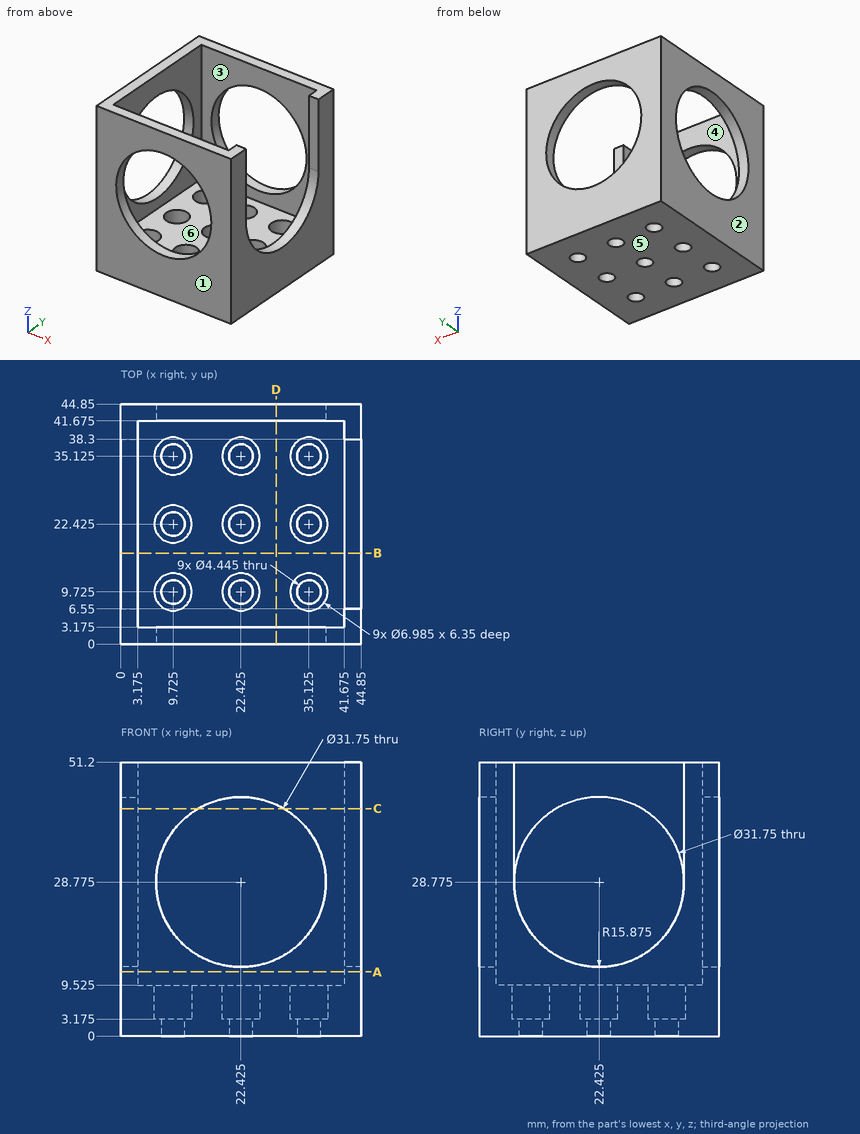
Geometry check sheet. Reference: drawing and pictorial views, mm from the part's lowest x, y, z. A direction names the side the tool comes from. Round coordinates to 2 decimals unless told otherwise and drop trailing zeros. Loops run counter-clockwise (first coordinate to the right, second up) from the corner with the lowest first, then second, coordinate; pieces in that order, holes last. Notation, with made-up numbers: (66.5, 68) - (124.5, 68) arc R36 cw to (124.5, 104) - close; hole circle Ø2 at (6, 33.25). An arc over 180 degrees is marked (long way). Use a Markdown table: item, result.
Q1. Access from +Z, -Z, +X, -X, +Y, -Y to the whole of each face (thin tool, end or side, straight path). Record for the marked faces 5 and 6.
Solutions:
| item | result |
|---|---|
| face 5 | -Z, +X, -X, +Y, -Y |
| face 6 | +Z |
Q2. Cross-section at C-C on z = 42.5. Record the cut outline in (x, y) (3 decimals), plus the area to 3 significant figures.
Solutions:
| item | result |
|---|---|
| outline | (0, 0) - (14.448, 0) - (14.448, 3.175) - (3.175, 3.175) - (3.175, 14.448) - (0, 14.448) - close; (0, 30.402) - (3.175, 30.402) - (3.175, 41.675) - (14.448, 41.675) - (14.448, 44.85) - (0, 44.85) - close; (30.402, 0) - (44.85, 0) - (44.85, 6.55) - (41.675, 6.55) - (41.675, 3.175) - (30.402, 3.175) - close; (30.402, 41.675) - (41.675, 41.675) - (41.675, 38.3) - (44.85, 38.3) - (44.85, 44.85) - (30.402, 44.85) - close |
| area | 276 mm2 |
Q3. Cross-section at D-D on x = 29. Record the cut outline in (y, z) (3 decimals), plus the area to 3 significant figures.
Solutions:
| item | result |
|---|---|
| outline | (0, 0) - (44.85, 0) - (44.85, 14.326) - (41.675, 14.326) - (41.675, 9.525) - (3.175, 9.525) - (3.175, 14.326) - (0, 14.326) - close; (0, 43.224) - (3.175, 43.224) - (3.175, 51.2) - (0, 51.2) - close; (41.675, 43.224) - (44.85, 43.224) - (44.85, 51.2) - (41.675, 51.2) - close |
| area | 508 mm2 |
Q4. Draft check along Y on the marked faces 1, 2, 3 and 4. Enter one of: released by +Y, released by -Y, zero draft, split by the parting line, or undercut.
Solutions:
| item | result |
|---|---|
| face 1 | released by -Y |
| face 2 | zero draft |
| face 3 | undercut |
| face 4 | undercut |
Q5. Cross-section at B-B on y = 17. Record the cut outline in (x, z) (3 decimals).
Solutions:
| item | result |
|---|---|
| outline | (0, 0) - (44.85, 0) - (44.85, 13.856) - (41.675, 13.856) - (41.675, 9.525) - (3.175, 9.525) - (3.175, 13.856) - (0, 13.856) - close; (0, 43.694) - (3.175, 43.694) - (3.175, 51.2) - (0, 51.2) - close |
Q6. Material ranges on line 1 (Y direction, x = 19, z = 12) (3 decimals); line 2 (X direction, y = 34, z = 3.5), recorded low to high.
Solutions:
| item | result |
|---|---|
| line 1 | y = 0 to 3.175, 41.675 to 44.85 |
| line 2 | x = 0 to 6.42, 13.03 to 19.12, 25.73 to 31.82, 38.43 to 44.85 |
Q7. Go/stop test with flat-tipped pins: P1, Ø6.5, axis at x = 22.425, y = 9.725, coming from the +Z side (3 decimals); P2, Ø7.5, axis at x = 33.5, y = 34.5, coming from the +Z side (3 decimals). Record where each tip stops, or that it passes through.
Solutions:
| item | result |
|---|---|
| P1 | stops at z = 3.175 |
| P2 | stops at z = 9.525 |
Q8. Cross-section at A-A on z = 12. Record the cut outline in (x, y) (3 decimals), plus the area to 3 significant figures.
Solutions:
| item | result |
|---|---|
| outline | (0, 0) - (44.85, 0) - (44.85, 44.85) - (0, 44.85) - close; hole (3.175, 3.175) - (41.675, 3.175) - (41.675, 41.675) - (3.175, 41.675) - close |
| area | 529 mm2 |
